Design review of the part shown in the three views and the two pictorial views. Dimensions are in mm from the part's minimum x, y and z. Coordinates: 2 decimals unless noted, no trailing zeros. Loops run counter-clockwise (first coordinate to the right, second up) from the corner with the lowest first, then second, coordinate; pieces in that order, holes last.
Q1. For P1, Ø3, axis at y = 3, z = 17, coming from the -X side; P2, Ø2, axis at y = 3, z = 17.5, coming from the -X side; P3, Ø11, axis at x = 12.5, z = 12.5, coming from the -Y side (3 decimals); P4, Ø2, axis at y = 3.5, z = 22.5, coming from the +X side, all flat-tipped, find the tip position at first contact; note any pin that passes through.
Q2. Wall thickness on probe 1 along Z at (x, y) = (12.5, 2.4); probe 2 along Y at (x, z) = (23.25, 16.75) (3 decimals): over which ranges is each line inside the solid? List them lowest first.
Q3. Add section B-B on y = 3.7. Give the boundary of the cut face in (x, z).
Q4. Draft analysis for pull direction Z (two halves, no side actions). For the marked faces 1, 2 and 3, state which applies: released by +Z, released by -Z, zero draft, split by the parting line, or undercut.
Q5. Add section C-C on y = 1. Give the boundary of the cut face in (x, z).
Q6. Add section A-A on z = 12.5. Give the boundary of the cut face in (x, y) (3 decimals), and give its area (3 significant figures).
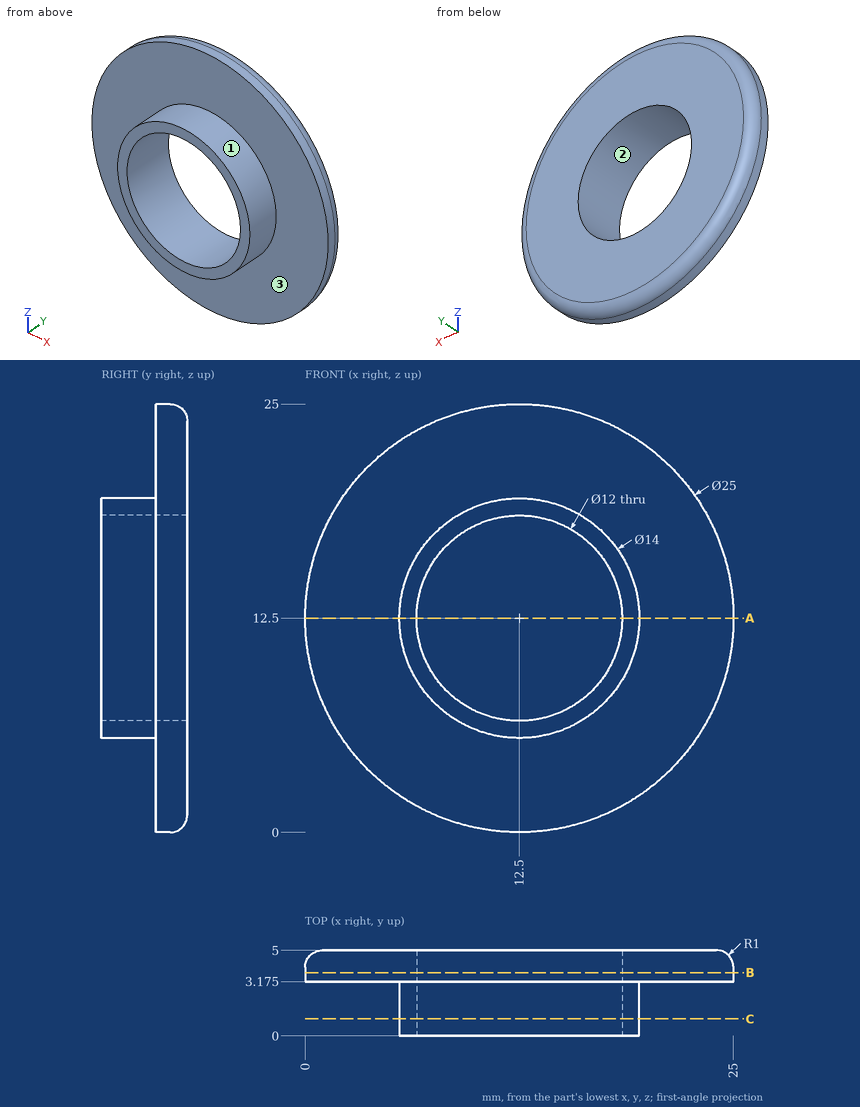
Entries:
1. P1: stops at x = 0.37
1. P2: stops at x = 0.66
1. P3: passes through
1. P4: stops at x = 21.17
2. probe 1: z = 5.5 to 6.5, 18.5 to 19.5
2. probe 2: y = 3.175 to 4.998
3. outline: circle Ø25 at (12.5, 12.5); hole circle Ø12 at (12.5, 12.5)
4. face 1: split by the parting line
4. face 2: undercut
4. face 3: zero draft
5. outline: circle Ø14 at (12.5, 12.5); hole circle Ø12 at (12.5, 12.5)
6. outline: (0, 3.175) - (5.5, 3.175) - (5.5, 0) - (6.5, 0) - (6.5, 5) - (1, 5) arc R1 ccw to (0, 4) - close; (18.5, 0) - (19.5, 0) - (19.5, 3.175) - (25, 3.175) - (25, 4) arc R1 ccw to (24, 5) - (18.5, 5) - close
6. area: 29.6 mm2
